Autodesk Inventor part; units mm, degrees
ref_plane "Work Plane2" through (4.456703, -9.721274, 3.970957) normal (0, 0, -1) x (0.4305111, 0.9025853, 0)
ref_plane "YZ Plane" through (0, 0, 0) normal (1, 0, 0) x (0, 1, 0)
ref_plane "XZ Plane" through (0, 0, 0) normal (0, 1, 0) x (-1, 0, 0)
ref_plane "Work Plane1" through (0, 0, 1.5) normal (0, 0, 1) x (1, 0, 0)
sketch "Sketch1" plane through (0, 0, 1.5) normal (0, 0, 1) x (1, 0, 0)
  line L0 (8.75354, 57.756452) -> (7.809034, 57.756452) construction
  line L1 (-24.776894, -15.05709) -> (8.75354, 57.756452) construction
  line L2 (-24.776894, -52.66184) -> (-24.776894, -15.05709) construction
  line L3 (-18.707308, -55.556884) -> (-24.776894, -52.66184) construction
  line L4 (-18.707308, -40.563421) -> (-18.707308, -55.556884) construction
  line L5 (0.391621, -40.563421) -> (-18.707308, -40.563421) construction
  line L6 (23.692692, 8.28829) -> (0.391621, -40.563421) construction
  line L7 (23.692692, 53.178978) -> (23.692692, 8.28829) construction
  line L8 (8.974225, 60.199326) -> (23.692692, 53.178978) construction
  line L9 (7.809034, 57.756452) -> (8.974225, 60.199326) construction
  circle A0 centre (-21.307308, -37.886297) radius 1.6 construction
  circle A1 centre (-21.307308, -27.886297) radius 1.6 construction
  line L10 (11.632256, -10.582296) -> (32.395806, 32.949392)
  line L11 (-15.355044, 2.289986) -> (5.408506, 45.821674)
  line L12 (5.408506, 45.821674) -> (32.395806, 32.949392)
  line L13 (32.395806, 32.949392) -> (-10.655303, -57.309136)
  line L14 (-10.655303, -57.309136) -> (-37.642603, -44.436855)
  line L15 (-37.642603, -44.436855) -> (5.408506, 45.821674)
  circle A2 centre (11.737087, 5.432666) radius 3
  circle A3 centre (-13.983408, -29.560487) radius 3
  circle A4 centre (-2.975053, 12.449997) radius 3
  point P0 (0, 0)
  dimension "d1" = 100
ref_plane "Work Plane2" through (4.456703, -9.721274, 3.970957) normal (0, 0, -1) x (0.4305111, 0.9025853, 0)
ref_plane "Work Plane6" through (4.456703, -9.721274, 2.470957) normal (0, 0, -1) x (0.4305111, 0.9025853, 0)
extrude "Extrusion1" add sketch "Sketch1" along normal up to surface (2.470957 mm away) contours L13 L14 L15 L11 L12 L10 | A2 | A3 | A4
sketch "Sketch2" plane through (-10.655303, -57.309136, 3.970957) normal (0, 0, 1) x (0.9025853, -0.4305111, 0)
  line L0 (0, 0) -> (0, 100)
  line L1 (0, 100) -> (-29.9, 100)
  line L2 (-29.9, 100) -> (-29.9, 0)
  line L3 (-29.9, 0) -> (0, 0)
  line L4 (-21.95, 51.77) -> (-27.9, 51.77)
  line L5 (-2, 51.77) -> (-7.95, 51.77)
  line L6 (-19.05, 34.77) -> (-10.85, 34.77)
  arc A0 (-27.45, 2.77) -> (-2.45, 2.77) centre (-14.95, 20.30125) ccw construction
  arc A1 (-2.45, 4.77) -> (-27.45, 4.77) centre (-14.95, -12.76125) ccw construction
  line L7 (-27.45, 2.77) -> (-27.45, 4.77) construction
  line L8 (-2.45, 2.77) -> (-2.45, 4.77) construction
  line L9 (-29.9, 0) -> (0, 0)
  line L10 (-25.477276, 0) -> (-25.477276, 7.745132)
  line L11 (-25.477276, 7.745132) -> (-16.899837, 31.078166)
  line L12 (-16.899837, 31.078166) -> (-16.899837, 41.065184)
  line L13 (-16.899837, 41.065184) -> (-29.9, 41.24513)
  line L14 (-29.9, 100) -> (-29.9, 0)
  line L15 (-29.9, 0) -> (-29.9, 41.24513)
  line L16 (-14.95, 0) -> (-14.95, 40.435372) construction
  line L17 (-2.45, 2.77) -> (-2.45, 4.77) construction
  line L18 (-4.422724, 0) -> (-4.422724, 7.745132)
  line L19 (-4.422724, 7.745132) -> (-13.000163, 31.078166)
  line L20 (-13.000163, 31.078166) -> (-13.000163, 41.065184)
  line L21 (-13.000163, 41.065184) -> (0, 41.24513)
  line L22 (0, 0) -> (0, 41.24513)
  line L23 (0, 0) -> (0, 100) construction
  line L24 (0, 41.24513) -> (0, 0) construction
  line L25 (0, 0) -> (-4.422724, 0) construction
  point P0 (-15.054899, 56.31361)
extrude "Extrusion2" add sketch "Sketch2" along normal blind 16 contours L3 L2 L13 L12 L11 L10
ref_plane "Work Plane3" through (-24.148953, -50.872995, 3.970957) normal (0.9025853, -0.4305111, 0) x (0, 0, -1)
mirror "Mirror1" about plane through (-24.148953, -50.872995, 3.970957) normal (0.9025853, -0.4305111, 0) of "Extrusion2"
sketch "Sketch3" plane through (-4.710042, -14.647591, 19.970957) normal (0.4179776, 0.9084573, 0) x (0.9084573, -0.4179776, 0)
  ellipse E0 centre (-1.967577, -0.95) end of major axis (-1.967577, 1.897221) minor radius 2.846948 construction
  line L0 (2.132031, -4.8) -> (2.132031, 2.9) construction
  line L1 (2.132031, 2.9) -> (-6.067184, 2.9) construction
  line L2 (-6.067184, 2.9) -> (-6.067184, -4.8) construction
  line L3 (-6.067184, -4.8) -> (2.132031, -4.8) construction
  line L4 (2.132031, -4.8) -> (2.132031, 2.9)
  line L5 (2.132031, 2.9) -> (-6.067184, 2.9)
  line L6 (-6.067184, 2.9) -> (-6.067184, -4.8)
  line L7 (-6.067184, -4.8) -> (2.132031, -4.8)
  line L8 (2.132031, 2.9) -> (-6.067184, 2.9)
  line L9 (-6.067184, 2.9) -> (-6.067184, 3.9)
  line L10 (-6.067184, 3.9) -> (2.132031, 3.9)
  line L11 (2.132031, 3.9) -> (2.132031, 2.9)
  ellipse E1 centre (-2.037491, 0.97324) end of major axis (-2.037491, 3.820462) minor radius 2.846948
  line L12 (2.062116, -2.87676) -> (2.062116, 4.82324)
  line L13 (-6.137098, -2.87676) -> (2.062116, -2.87676)
  line L14 (-6.137098, 4.82324) -> (-6.137098, -2.87676)
  line L15 (2.062116, 4.82324) -> (-6.137098, 4.82324)
  point P0 (-1.843493, 19.970957)
  dimension "d6" = 0
  dimension "d40" = 1
extrude "Extrusion3" cut sketch "Sketch3" along normal through all both and the other way through all contours L5 L12 L10 L11 | L12 L13 L6 L5 E1 | L5 E1 L9 L10 L12 | L13 L14 L15 L12 L10 L9 L6 | E1 L5 | L5 E1
sketch "Sketch4" plane through (-24.148953, -50.872995, 3.970957) normal (0.9025853, -0.4305111, 0) x (0, 0, -1)
  arc A0 (-27.45, 2.77) -> (-2.45, 2.77) centre (-14.95, 20.30125) ccw
  line L0 (-27.45, 2.77) -> (-27.45, 4.77)
  arc A1 (-2.45, 4.77) -> (-27.45, 4.77) centre (-14.95, -12.76125) ccw
  arc A2 (-2.475103, 4.91042) -> (-27.55, 4.82144) centre (-14.95, -12.76125) ccw
  line L1 (-27.55, 4.82144) -> (-27.55, 2.71856)
  arc A3 (-27.55, 2.71856) -> (-2.475103, 2.62958) centre (-14.95, 20.30125) ccw
  line L2 (-15.02676, 8.869864) -> (-15.02676, -1.329864)
  point P0 (3.970957, 56.31361)
  dimension "d9" = 0.1
revolve "Revolution1" cut sketch "Sketch4" angle 360 about axis through (-20.330379, -42.867187, 18.997716) along (-0.4305111, -0.9025853, 0)
sketch "Sketch5" plane through (0, 0, 1.5) normal (0, 0, -1) x (-1, 0, 0)
  circle A0 centre (-11.737087, 5.432666) radius 3 construction
  circle A1 centre (2.975053, 12.449997) radius 3 construction
  point P0 (0, 0)
sketch "Sketch6" plane through (0, 0, 1.5) normal (0, 0, -1) x (-1, 0, 0)
  line L0 (-4.381017, 8.941331) -> (-7.825106, 16.162014)
  line L1 (-8.686128, 17.967184) -> (-12.130217, 25.187866)
  circle A0 centre (10.53932, -22.339805) radius 2.45
  circle A1 centre (-15.181176, 12.653348) radius 2.45
  circle A2 centre (-0.469036, 19.670679) radius 2.45
  circle A3 centre (-7.285825, -3.551175) radius 1.45
  circle A4 centre (7.155539, 3.337003) radius 1.45
  line L2 (-32.395806, 32.949392) -> (-5.408506, 45.821674)
  line L3 (10.655303, -57.309136) -> (-32.395806, 32.949392)
  point P0 (0, 0)
  dimension "d48" = 8
  dimension "d51" = 4.9
  dimension "d54" = 4.9
  dimension "d55" = 4.9
  dimension "d56" = 2.9
  dimension "d57" = 2.9
  dimension "d83" = 43.755
  dimension "d84" = 43.755
  dimension "d85" = 13.1
  dimension "d86" = 6.95
sketch "Sketch7" plane through (5.408506, 45.821674, 3.970957) normal (0, 0, 1) x (0.9025853, -0.4305111, 0)
  line L0 (25.477276, -100) -> (25.477276, -92.254868)
  line L1 (25.477276, -92.254868) -> (16.899837, -68.921834)
  line L2 (16.899837, -68.921834) -> (16.899837, -58.934816)
  line L3 (16.899837, -58.934816) -> (29.9, -58.75487)
  line L4 (29.9, -58.75487) -> (29.9, 0)
  line L5 (29.9, 0) -> (0, 0)
  line L6 (0, 0) -> (0, -58.75487)
  line L7 (0, -58.75487) -> (13.000163, -58.934816)
  line L8 (13.000163, -58.934816) -> (13.000163, -68.921834)
  line L9 (13.000163, -68.921834) -> (4.422724, -92.254868)
  line L10 (4.422724, -92.254868) -> (4.422724, -100)
  line L11 (4.422724, -100) -> (25.477276, -100)
  line L12 (13.000163, -58.934816) -> (13.000163, -68.921834)
  line L13 (13.000163, -58.934816) -> (16.899837, -58.934816)
  point P0 (14.845101, -43.68639)
extrude "Extrusion5" add sketch "Sketch7" along normal blind 2
sketch "Sketch8" plane through (32.395806, 32.949392, 3.970957) normal (0.9025853, -0.4305111, 0) x (0, 0, -1)
  line L0 (2.470957, -100) -> (-16, -100)
  line L1 (2.470957, -100) -> (2.470957, 0)
  line L2 (-2, -58.75487) -> (-16, -58.75487)
  line L3 (-16, -58.75487) -> (-16, -100)
  line L4 (-16, -100) -> (2.470957, -100)
  line L5 (2.470957, -100) -> (2.470957, 0)
  line L6 (2.470957, 0) -> (-16, 0)
  line L7 (-16, 0) -> (-16, -100)
  line L8 (2.470957, 0) -> (-2, 0)
  line L9 (-2, -58.75487) -> (-2, 0)
  line L10 (-16, -58.75487) -> (2.470957, -58.75487)
  line L11 (2.470957, -100) -> (2.470957, 0)
  point P0 (3.970957, -43.68639)
extrude "Extrusion7" add sketch "Sketch8" along normal blind 1.05 contours L0 L3 L2 L10 L1 | L10 L9 L6 L1
ref_plane "Work Plane4" through (-74.107308, 67.113703, 4) normal (0, 1, 0) x (1, 0, 0)
sketch "Sketch10" plane through (-74.107308, 67.113703, 4) normal (0, 1, 0) x (1, 0, 0)
  circle A0 centre (-42.022145, 16.72324) radius 3
  circle A1 centre (-42.022145, 16.72324) radius 4.301236
  point P0 (74.107308, 4)
extrude "Extrusion9" cut sketch "Sketch10" against normal through all contours A0 | A1
ref_plane "Work Plane5" through (0, 0, 0) normal (0, 0, -1) x (-1, 0, 0)
sketch "Sketch12" plane through (-24.148953, -50.872995, 3.970957) normal (0.9025853, -0.4305111, 0) x (0, 0, -1)
  line L0 (-25.02676, 14.71856) -> (-5.02676, 14.71856)
  line L1 (-25.02676, 14.71856) -> (-25.02676, 13.31856)
  arc A0 (-25.02676, 13.31856) -> (-15.093782, 10.018425) centre (-15.093782, 26.616977) ccw
  line L2 (-5.02676, 14.81856) -> (-25.12676, 14.81856)
  line L3 (-25.12676, 14.81856) -> (-25.12676, 13.268531)
  arc A1 (-25.12676, 13.268531) -> (-15.093782, 9.918425) centre (-15.093782, 26.616977) ccw
  line L4 (-15.093782, 9.918425) -> (-15.093782, 14.81856)
  line L5 (-15.093782, 9.918425) -> (-10.193647, 9.918425) construction
  point P0 (3.970957, 56.31361)
  dimension "d41" = 0.1
  dimension "d42" = 90
revolve "Revolution2" cut sketch "Sketch12" angle 360 about axis through (-19.878961, -41.920771, 19.064739) along (0.4305111, 0.9025853, 0)
sketch "Sketch13" plane through (33.343521, 32.497355, 3.970957) normal (0.9025853, -0.4305111, 0) x (0, 0, -1)
  line L0 (2.470957, -100) -> (-16, -100)
  line L1 (-16, 0) -> (-16, -100)
  line L2 (3.970957, -100) -> (-16, -100)
  line L3 (-16, -100) -> (-16, -91)
  line L4 (-16, -91) -> (3.970957, -91)
  line L5 (3.970957, -91) -> (3.970957, -100)
  point P0 (3.970957, -43.68639)
  dimension "d44" = 9
extrude "Extrusion10" cut sketch "Sketch13" against normal through all
hole "Hole3" at (7.285825, -3.551175, 1.5) at (-7.155539, 3.337003, 1.5) direction (0, 0, 1) diameter 2.9 end through all counterbore diameter 6 counterbore depth 0.5
sketch "Sketch14" plane through (0, 0, 1.5) normal (0, 0, -1) x (-1, 0, 0)
  circle A0 centre (9.333775, -19.812328) radius 2.45
  circle A1 centre (-16.38672, 15.180825) radius 2.45
  circle A2 centre (-1.67458, 22.198156) radius 2.45
  circle A3 centre (-19.486287, 21.679201) radius 1.45
  circle A4 centre (-4.774147, 28.696532) radius 1.45
  line L0 (29.359754, -38.416214) -> (11.188953, -47.083242)
  line L1 (20.274354, -42.749728) -> (9.333775, -19.812328)
  line L2 (-7.825106, 16.162014) -> (-8.600026, 17.786667)
  line L3 (-15.956209, 14.27824) -> (-1.243956, 21.295333)
  point P0 (0, 0)
  point P1 (0, 0)
  dimension "d73" = 4.9
  dimension "d74" = 4.9
  dimension "d75" = 4.9
  dimension "d76" = 2.9
  dimension "d77" = 2.9
  dimension "d94" = 25.413
  dimension "d95" = 1.8
extrude "Extrusion11" cut sketch "Sketch14" against normal blind 4.471 contours A0 | A1 | A2
sketch "Sketch15" plane through (5.408506, 45.821674, 5.970957) normal (0, 0, 1) x (0.9025853, -0.4305111, 0)
  line L0 (13.000163, -58.934816) -> (13.000163, -68.921834)
  line L1 (4.884025, -91) -> (25.015975, -91)
  line L2 (16.899837, -68.921834) -> (25.015975, -91)
  line L3 (12.77916, -69.523024) -> (13.000163, -68.921834)
  line L4 (4.884025, -91) -> (13.000163, -68.921834)
  line L5 (29.9, -58.75487) -> (16.899837, -58.934816)
  line L6 (13.000163, -58.934816) -> (16.899837, -58.934816)
  line L7 (16.899837, -68.921834) -> (16.899837, -58.934816)
  line L8 (17.12084, -69.523024) -> (16.899837, -68.921834)
  point P0 (14.845101, -43.68639)
extrude "Extrusion12" add sketch "Sketch15" along normal blind 2
sketch "Sketch16" plane through (-19.886117, -7.209607, 5.970957) normal (-0.9025853, 0.4305111, 0) x (0, 0, 1)
  line L0 (-4.470957, -32.24513) -> (14, -32.24513)
  line L1 (14, 0) -> (14, -32.24513)
  line L2 (0, 0) -> (14, 0)
  line L3 (0, 58.75487) -> (0, 0)
  line L4 (-4.470957, 58.75487) -> (0, 58.75487)
  line L5 (-4.470957, 58.75487) -> (-4.470957, -32.24513)
  point P0 (-5.970957, 15.068479)
extrude "Extrusion13" add sketch "Sketch16" along normal blind 1.05
sketch "Sketch17" plane through (33.343521, 32.497355, 3.970957) normal (0.9025853, -0.4305111, 0) x (0, 0, -1)
  line L0 (2.470957, 0) -> (-2, 0)
  line L1 (2.470957, 0) -> (2.470957, -91)
  line L2 (-2, 0) -> (2.470957, 0)
  line L3 (2.470957, 0) -> (2.470957, -10.755)
  line L4 (2.470957, -10.755) -> (-2, -10.755)
  line L5 (-2, -10.755) -> (-2, 0)
  point P0 (3.970957, -43.68639)
  dimension "d89" = 10.755
extrude "Extrusion14" cut sketch "Sketch17" against normal through all
properties part number "30_CUBE_openSIM_Laser_Telescope_Mount"
The model under review builds one solid part; all positions refer to its coordinate system, in mm. A direction names the side the tool comes from. Coordinates: 2 decimals unless noted, no trailing zeros. Loops run counter-clockwise (first coordinate to the right, second up) from the corner with the lowest first, then second, coordinate; pieces in that order, holes last. Notation, with made-up numbers: (80, 1.25) -> (139, 1.25) arc R5 cw to (139, 7.25) -> close; hole circle Ø2 at (89.25, 71). An arc over 180 degrees is marked (long way). Answer as CSV lines item,"result".
Item 1: Take a section at D-D, the plane y = -32. State the section outline as (x, z) points.
Results below:
outline,"(-32.87, 1.5) -> (2.58, 1.5) -> (2.58, 19.97) -> (-9.79, 19.97) -> (-9.79, 7.97) -> (-22.79, 7.97) -> (-22.79, 19.97) -> (-32.87, 19.97) -> close"
Item 2: Take a section at B-B, the plane y = 14. State the section outline as (x, z) points.
Results below:
outline,"(-10.93, 1.5) -> (14.24, 1.5) -> (14.24, 5.97) -> (-10.93, 5.97) -> close; (18.53, 1.5) -> (24.52, 1.5) -> (24.52, 5.97) -> (18.53, 5.97) -> close"
Item 3: Take a section at A-A, the plane z = 10.75. State the section outline as (x, y) points, and give its area (3 significant figures).
Results below:
outline,"(-34.72, -35.86) -> (-29.36, -38.42) -> (-12.53, -21.98) -> (-8.23, -12.97) -> (-19.89, -7.21) -> (-20.83, -6.76) -> close; (-11.19, -47.08) -> (-5.83, -49.64) -> (8.05, -20.53) -> (7.1, -20.08) -> (-4.71, -14.65) -> (-9.01, -23.66) -> close"
area,"725 mm2"
Item 4: Draft analysis for pull direction X (two halves, no side actions). For faces 6 (the flat face through (-6.49, -13.8, 6.96)), 7 (the flat face through (-3, -6, 1.5)), 8 (the cylindrical face through (-8.803, -22.204, 3.704)), state which applies: +X half, -X half, draft (parallel to the pull), parting line (faces both ways), or undercut.
Results below:
face 6,"+X half"
face 7,"draft"
face 8,"undercut"
Item 5: For L1, parallel to X at y = -37, z = 14.5; L2, parallel to Z at x = -3.5, y = -0.5; L3, parallel to Z at x = -7, y = -24, list the stretches that pass through material, from the lowest coordinate up.
Results below:
L1,"x = -32.33 to -27.91, -10.25 to 0.19"
L2,"z = 1.5 to 5.97"
L3,"z = 1.5 to 15.15"
Item 6: Take a section at C-C, the plane z = 3.75. State the section outline as (x, y) points, and give its area (3 significant figures).
Results below:
outline,"(-34.72, -35.86) -> (-5.83, -49.64) -> (28.71, 22.79) -> (-0.17, 36.57) -> close; hole circle Ø4.9 at (-9.33, -19.81); hole circle Ø2.9 at (-7.16, 3.34); hole circle Ø4.9 at (1.67, 22.2); hole circle Ø2.9 at (7.29, -3.55); hole circle Ø4.9 at (16.39, 15.18)"
area,"2,500 mm2"
Item 7: Machinability: for faces 1 (the flat face through (-16, -34, 7.971)), 2 (the flat face through (-7, -21, 15.148)), 3 (the flat face through (9, -4, 2)), 4 (the flat face through (-13.976, -10.129, 12.873)), 5 (the flat face through (-6.256, -23.109, 16.564)), which of the approach directions +Z, -Z, +X, -X, +Y, -Y give a long, thin tool a straight path to every point of the face, cutting with its end or side? Answer none if there is none.
Results below:
face 1,"+Z"
face 2,"+Z, +Y"
face 3,"-Z"
face 4,"+Z, +X, +Y"
face 5,"+Y"
Item 8: Insertion check: pin 1 (2 mm diameter, centred on y = 8.5, z = 8, fed in from +X); pin 2 (0.7 mm diameter, centred on x = -7.5, y = -20.5, fed in from -Z); pin 3 (1.5 mm diameter, centred on x = -11.5, y = 13, fed in from +Z); pin 4 (4 mm diameter, centred on x = 3, z = 13, fed in from -Y). Each pin has a flat end and moves straight along its axis. Give the tip position at first contact, or say it passes through.
Results below:
pin 1,"passes through"
pin 2,"stops at z = 5.97"
pin 3,"stops at z = 5.97"
pin 4,"stops at y = -35.31"
